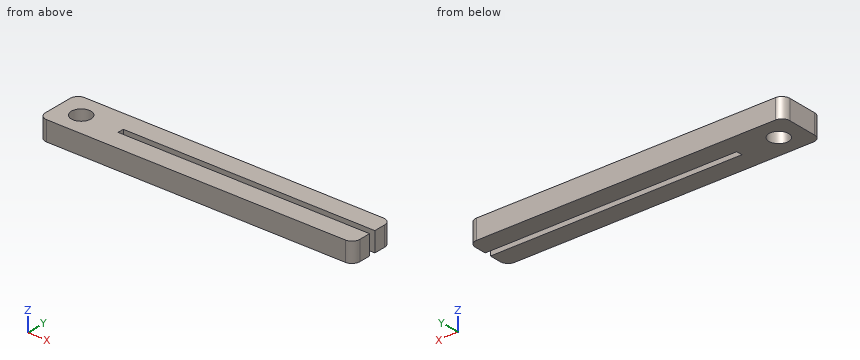
Autodesk Inventor part; units mm, degrees
ref_plane "YZ Plane" through (0, 0, 0) normal (1, 0, 0) x (0, 1, 0)
ref_plane "XZ Plane" through (0, 0, 0) normal (0, 1, 0) x (-1, 0, 0)
ref_plane "XY Plane" through (0, 0, 0) normal (0, 0, 1) x (1, 0, 0)
sketch "Эскиз1" plane through (0, 0, 0) normal (0, 1, 0) x (-1, 0, 0)
  point P0 (0, 0)
sketch "Эскиз2" plane through (0, 0, 0) normal (0, 0, 1) x (1, 0, 0)
  line L0 (0, 0) -> (80, 0)
  line L1 (80, 0) -> (80, 5)
  line L2 (80, 5) -> (0, 5)
  line L3 (0, 5) -> (0, 0)
  line L4 (0, 5) -> (16, 5)
  line L5 (16, 5) -> (16, 6.6)
  line L6 (16, 6.6) -> (0, 6.6)
  line L7 (0, 6.6) -> (0, 5)
  line L8 (0, 6.6) -> (80, 6.6)
  line L9 (80, 6.6) -> (80, 11.6)
  line L10 (80, 11.6) -> (0, 11.6)
  line L11 (0, 11.6) -> (0, 6.6)
  dimension "d0" = 5
  dimension "d1" = 80
  dimension "d2" = 16
  dimension "d3" = 1.6
  dimension "d4" = 80
  dimension "d5" = 5
extrude "Выдавливание1" add sketch "Эскиз2" along normal blind 5
fillet "Сопряжение1" radius 2 4 edges at (0, 0, 2.5) (0, 11.6, 2.5) (80, 0, 2.5) (80, 11.6, 2.5)
sketch "Эскиз3" plane through (0, 0, 0) normal (0, 0, -1) x (-1, 0, 0)
  circle A0 centre (-6, 5.75) radius 2.5
  line L0 (-16, 5) -> (-16, 6.6)
  line L1 (-16, 5.75) -> (-16, 5)
  point P0 (0, 0)
  dimension "d9" = 5
extrude "Выдавливание2" cut sketch "Эскиз3" against normal blind 13.75
properties part number "Bush_phase_mono" material "Медь"
Read the model definition and answer for the solid it produces. Units are mm, in the model's axes. Give positions to 0.01 mm unless a question says otherwise; leave off trailing zeros. Write each loop counter-clockwise with the first axis right and the second up, starting at its lowest first coordinate (ties: lowest second). Pieces come first, ordered by that corner, then holes. Notation, with made-up numbers: (39.5, -36.75) -> (87.5, -36.75) arc R18 ccw to (87.5, -10.75) -> close; hole circle Ø6 at (75.25, 83.5). An arc over 180 degrees is marked (long way). Answer as a JSON object with one key per item and string values. Group by question number.
1) Consider L1, parallel to Y at x = 16.5, z = 3.9; L2, parallel to Y at x = 6, z = 1.45; L3, parallel to X at y = 3.5, z = 2.75. Determine where each line is inside the solid, lowest interval first. Write a range as from..to.
2) Find section A-A (x = 62). Write down the section's boundary in (y, z).
3) Find section C-C (y = 5.75). Write down the section's boundary in (x, z), and give its area (3 significant figures).
4) This flat-tipped pin is pushed along its axis until it touches: P1, Ø3, axis at x = 6, y = 5.75, coming from the +Z side. Where does it stop, or does it pass through?
5) Find section B-B (z = 1.4). Write down the section's boundary in (x, y), and give its area (3 significant figures).
Values follow:
{
 "1": {"L1": "y = 0..5, 6.6..11.6", "L2": "y = 0..3.25, 8.25..11.6", "L3": "x = 0..4.91, 7.09..80"},
 "2": {"outline": "(0, 0) -> (5, 0) -> (5, 5) -> (0, 5) -> close; (6.6, 0) -> (11.6, 0) -> (11.6, 5) -> (6.6, 5) -> close"},
 "3": {"outline": "(0, 0) -> (3.5, 0) -> (3.5, 5) -> (0, 5) -> close; (8.5, 0) -> (16, 0) -> (16, 5) -> (8.5, 5) -> close", "area": "55.0 mm2"},
 "4": {"P1": "passes through"},
 "5": {"outline": "(0, 2) arc R2 ccw to (2, 0) -> (78, 0) arc R2 ccw to (80, 2) -> (80, 5) -> (16, 5) -> (16, 6.6) -> (80, 6.6) -> (80, 9.6) arc R2 ccw to (78, 11.6) -> (2, 11.6) arc R2 ccw to (0, 9.6) -> close; hole circle Ø5 at (6, 5.75)", "area": "803 mm2"}
}
